Read the model definition and answer for the solid it produces. Units are mm, in the model's axes. A direction names the side the tool comes from. Round coordinates to 2 decimals unless told otherwise and drop trailing zeros. Order: outer loops, then holes, each group sorted by start corner. A loop starts at its lowest first (then second) coordinate and runs counter-clockwise, first axis right, second up. Notation, with made-up numbers: M 3.25,18.25 L 25.25,18.25 A17 cw 25.25,32.25 Z; hole C -14,-6 d3. An arc over 180 degrees is marked long. Answer as CSV lines item,"result".
```python
from build123d import *

# Parameters (mm, degrees)
F0_R     = 15
F1_DEPTH = 2
F3_DEPTH = 2.001
F5_DEPTH = 0.25
F6_R     = 12.5
F7_DEPTH = 0.25


with BuildPart() as f1:
    # F0 (on Front) → F1 (new body)
    with BuildSketch(Plane.XZ):
        with BuildLine():
            Line((74.7654586344, 19.9989924685), (-75.0312126981, 19.9989924685))
            ThreePointArc((-75.0312126981, 19.9989924685), (-95.2302513379, -0.261571778), (-74.5082089138, -19.9869002501))
            Line((-74.5082089138, -19.9869002501), (-8.7254105168, -19.9869002501))
            ThreePointArc((-8.7254105168, -19.9869002501), (-4.839616653, -19.2010527368), (-1.5645510783, -16.9670214598))
            Line((-1.5645510783, -16.9670214598), (13.5023982574, -1.5099393951))
            ThreePointArc((13.5023982574, -1.5099393951), (15.1399310448, -0.3929237566), (17.0828279766, 0))
            Line((17.0828279766, 0), (20.6616625341, 0))
            ThreePointArc((20.6616625341, 0), (23.6645705828, -1.0021826891), (25.4636936461, -3.6069826995))
            Line((25.4636936461, -3.6069826995), (29.2526781559, -16.6684295982))
            Line((29.2526781559, -16.6684295982), (33.0697437835, -3.5983243492))
            ThreePointArc((33.0697437835, -3.5983243492), (34.8699530038, -0.9994763934), (37.8692547347, 0))
            Line((37.8692547347, 0), (50.4326597146, 0))
            ThreePointArc((50.4326597146, 0), (53.3846342659, -0.9644273952), (55.1978227663, -3.4856615005))
            Line((55.1978227663, -3.4856615005), (56.8249496751, -8.6057353998))
            ThreePointArc((56.8249496751, -8.6057353998), (57.5502250753, -9.6142290419), (58.7310148958, -10))
            Line((58.7310148958, -10), (60.8050612923, -10))
            ThreePointArc((60.8050612923, -10), (61.9858511128, -9.6142290419), (62.711126513, -8.6057353998))
            Line((62.711126513, -8.6057353998), (65.3225235362, -0.3884625696))
            ThreePointArc((65.3225235362, -0.3884625696), (65.7154835042, -0.0469275173), (66.1990398413, -0.2398964195))
            Line((66.1990398413, -0.2398964195), (69.4730335519, -4.6052213669))
            ThreePointArc((69.4730335519, -4.6052213669), (69.7287348247, -4.8933610183), (70.0987919677, -5.0004372085))
            Line((70.0987919677, -5.0004372085), (70.7654586344, -5.0004372085))
            ThreePointArc((70.7654586344, -5.0004372085), (71.119012025, -4.8539905991), (71.2654586344, -4.5004372085))
            Line((71.2654586344, -4.5004372085), (71.2654586344, -4.0004372085))
            ThreePointArc((71.2654586344, -4.0004372085), (72.2654586344, -3.2196608021), (73.2654586344, -4.0004372085))
            Line((73.2654586344, -4.0004372085), (73.2654586344, -4.5004372085))
            ThreePointArc((73.2654586344, -4.5004372085), (73.4119052438, -4.8539905991), (73.7654586344, -5.0004372085))
            Line((73.7654586344, -5.0004372085), (74.2654586344, -5.0004372085))
            ThreePointArc((74.2654586344, -5.0004372085), (74.7126722299, -4.8948643995), (75.0654586344, -4.6004372085))
            Line((75.0654586344, -4.6004372085), (78.3864482289, -0.1724510824))
            ThreePointArc((78.3864482289, -0.1724510824), (78.5628414312, -0.0252374869), (78.7864482289, 0.0275489176))
            Line((78.7864482289, 0.0275489176), (79.7654586344, 0.0275489176))
            ThreePointArc((79.7654586344, 0.0275489176), (83.3009925403, 1.4920150116), (84.7654586344, 5.0275489176))
            Line((84.7654586344, 5.0275489176), (84.7654586344, 9.9989924685))
            ThreePointArc((84.7654586344, 9.9989924685), (81.8365264462, 17.0700602804), (74.7654586344, 19.9989924685))
        make_face()
        with Locations((-75.231961906, 0)):
            Circle(F0_R, mode=Mode.SUBTRACT)
    extrude(amount=F1_DEPTH)

    # F2 (on Front) → F3 (cut, through all)
    with BuildSketch(Plane.XZ):
        with BuildLine():
            Line((-6.3686813228, -13.5), (-6.3686813228, 0))
            Line((-6.3686813228, 0), (-6.3686813228, 13.5))
            ThreePointArc((-6.3686813228, 13.5), (-14.9944197626, 15.137553477), (-23.3686813228, 12.5))
            Line((-23.3686813228, 12.5), (-23.3686813228, 8.413849912))
            ThreePointArc((-23.3686813228, 8.413849912), (-21.2785048492, 0), (-23.3686813228, -8.413849912))
            Line((-23.3686813228, -8.413849912), (-23.3686813228, -12.5))
            ThreePointArc((-23.3686813228, -12.5), (-14.9944197626, -15.137553477), (-6.3686813228, -13.5))
        make_face()
    extrude(amount=F3_DEPTH, mode=Mode.SUBTRACT)

    # F4 (on face) → F5 (cut)
    with BuildSketch(Plane.XZ.offset(2)):
        with BuildLine():
            Line((-23.3686813228, 8.413849912), (-23.3686813228, 9.2801801341))
            ThreePointArc((-23.3686813228, 9.2801801341), (-27.4944197626, 0), (-23.3686813228, -9.2801801341))
            Line((-23.3686813228, -9.2801801341), (-23.3686813228, -8.413849912))
            ThreePointArc((-23.3686813228, -8.413849912), (-21.2785048492, 0), (-23.3686813228, 8.413849912))
        make_face()
        with BuildLine():
            ThreePointArc((-6.3686813228, -9.046913085), (-3.5037337409, -4.9207859892), (-2.4944197626, 0))
            ThreePointArc((-2.4944197626, 0), (-3.5037337409, 4.9207859892), (-6.3686813228, 9.046913085))
            Line((-6.3686813228, 9.046913085), (-6.3686813228, -9.046913085))
        make_face()
    extrude(amount=-F5_DEPTH, mode=Mode.SUBTRACT)

    # F6 (on Front) → F7 (cut)
    with BuildSketch(Plane.XZ):
        with Locations((-14.9645612109, 0)):
            Circle(F6_R)
    extrude(amount=F7_DEPTH, mode=Mode.SUBTRACT)


solid = f1.part
```
Item 1: A cutting plane is placed at C-C, the plane x = -14.5. Determine the outline of the cut face in (y, z), and give its area (3 significant figures).
Ans:
outline,"M -2,-19.99 L 0,-19.99 L 0,-15.16 L -2,-15.16 Z; M -2,15.16 L 0,15.16 L 0,20 L -2,20 Z"
area,"19.3 mm2"
Item 2: Determine the mould class of faces 6 (the face through (81.914, -0.986, 16.992)), 7 (the face through (67.81, -0.99, -2.39)), 8 (the face through (-6, -2, 14)) for opening direction X: +X half, -X half, draft (parallel to the pull), parting line (faces both ways), or undercut.
Ans:
face 6,"+X half"
face 7,"undercut"
face 8,"draft"
Item 3: Flat-ended cylindrical pins translate along their axes: pin 1 (3 mm diameter, centred on x = 24, z = -6, fed in from +Y); pin 2 (0.8 mm diameter, centred on x = 79.5, y = -1, fed in from -Z); pin 3 (0.6 mm diameter, centred on y = -1, z = -10, fed in from +X); pin 4 (2 mm diameter, centred on x = -4.5, z = 0.5, fed in from +Y). Find the tip coordinate at first contact, or state that the pin passes through.
Ans:
pin 1,"through"
pin 2,"z = 0.03"
pin 3,"x = 61.86"
pin 4,"y = -0.25"
Item 4: A tool of negligible diameter and unlimited length cuts with its end or side. For faces 1 (the face through (-4.89, -0.99, -19.22)), 2 (the face through (-24, -0.25, 0)), 3 (the face through (53.35, -0.99, -0.94)), 4 (the face through (-90.217, -0.986, 0.66)), 5 (the face through (-5, -1.75, 0)), from which of +Z, -Z, +X, -X, +Y, -Y can it reach the whole face along a straight path? Write none if from no direction.
Ans:
face 1,"-Z, +X, +Y, -Y"
face 2,"+Y"
face 3,"-Z, +Y, -Y"
face 4,"+Y, -Y"
face 5,"-Y"
Item 5: Find the intervals of material crossed by probe 1 along X at (y, z) = (-1.1, 9.5); probe 2 along X at (y, z) = (-0.7, 10.5); probe 3 along Z at (x, y) = (-75.5, -0.3), in increasing order. Write a range as [from, to].
Ans:
probe 1,"[-92.83, -86.84], [-63.62, -23.37], [-6.37, 84.77]"
probe 2,"[-92.25, -85.94], [-64.52, -23.37], [-6.37, 84.75]"
probe 3,"[-20, -15], [15, 20]"
Item 6: A cutting plane is placed at D-D, the plane x = 11. Determine the outline of the cut face in (y, z), and give its area (3 significant figures).
Ans:
outline,"M -2,-4.08 L 0,-4.08 L 0,20 L -2,20 Z"
area,"48.2 mm2"
Item 7: A cutting plane is placed at B-B, the plane y = -1.3. Give the number of separate pieces and of enclosed holes in the cut face, and give its area (3 significant figures).
Ans:
separate pieces,"1"
enclosed holes,"2"
area,"4,440 mm2"
Item 8: A cutting plane is placed at A-A, the plane x = -83.5. Determine the outline of the cut face in (y, z), and give its area (3 significant figures).
Ans:
outline,"M -2,-18.21 L 0,-18.21 L 0,-12.52 L -2,-12.52 Z; M -2,12.52 L 0,12.52 L 0,18.21 L -2,18.21 Z"
area,"22.8 mm2"
